Part model, mm, in its own coordinate system. A direction names the side the tool comes from. Coordinates: 2 decimals unless noted, no trailing zeros. Write each loop counter-clockwise with the first axis right and the second up, starting at its lowest first coordinate (ties: lowest second). Pieces come first, ordered by that corner, then holes. Notation, with made-up numbers: (33, 49) -> (63, 49) arc R29 cw to (63, 83) -> close; hole circle Ø7 at (10.25, 2). An arc over 180 degrees is marked (long way). Write item = value, one per line.
from build123d import *

# Parameters (mm, degrees)
SKETCH1_R           = 19.05
SKETCH1_R_2         = 9.525
BOSS_EXTRUDE1_DEPTH = 136.3472
SKETCH2_R           = 1.7526
CUT_EXTRUDE1_DEPTH  = 9.525
SKETCH3_R           = 1.7526
CUT_EXTRUDE2_DEPTH  = 9.525
SKETCH6_R           = 11.1125
CUT_EXTRUDE3_DEPTH  = 5.55625
SKETCH7_R           = 11.1125
CUT_EXTRUDE4_DEPTH  = 5.55625


with BuildPart() as part:
    # Sketch1 → Boss-Extrude1 (new body)
    with BuildSketch(Plane.XY):
        Circle(SKETCH1_R)
        Circle(SKETCH1_R_2, mode=Mode.SUBTRACT)
    extrude(amount=BOSS_EXTRUDE1_DEPTH)

    # Sketch2 → Cut-Extrude1 (cut)
    with BuildSketch(Plane(origin=(0, 0, 0), x_dir=(-1, 0, 0), z_dir=(0, 0, -1))):
        with Locations((0, 15.24)):
            Circle(SKETCH2_R)
        with Locations((15.24, 0)):
            Circle(SKETCH2_R)
        with Locations((0, -15.24)):
            Circle(SKETCH2_R)
        with Locations((-15.24, 0)):
            Circle(SKETCH2_R)
    extrude(amount=-CUT_EXTRUDE1_DEPTH, mode=Mode.SUBTRACT)

    # Sketch3 → Cut-Extrude2 (cut)
    with BuildSketch(Plane.XY.offset(136.3472)):
        with Locations((0, 15.24)):
            Circle(SKETCH3_R)
        with Locations((15.24, 0)):
            Circle(SKETCH3_R)
        with Locations((0, -15.24)):
            Circle(SKETCH3_R)
        with Locations((-15.24, 0)):
            Circle(SKETCH3_R)
    extrude(amount=-CUT_EXTRUDE2_DEPTH, mode=Mode.SUBTRACT)

    # Sketch6 → Cut-Extrude3 (cut)
    with BuildSketch(Plane.XY.offset(136.3472)):
        Circle(SKETCH6_R)
    extrude(amount=-CUT_EXTRUDE3_DEPTH, mode=Mode.SUBTRACT)

    # Sketch7 → Cut-Extrude4 (cut)
    with BuildSketch(Plane(origin=(0, 0, 0), x_dir=(-1, 0, 0), z_dir=(0, 0, -1))):
        Circle(SKETCH7_R)
    extrude(amount=-CUT_EXTRUDE4_DEPTH, mode=Mode.SUBTRACT)


solid = part.part
Q1. Saw through at C-C on y = 15.24. Give the cut face in (x, z) (3 decimals), and give its area (3 significant figures).
Model answer:
outline = (-11.43, 0) -> (-1.753, 0) -> (-1.753, 9.525) -> (1.753, 9.525) -> (1.753, 0) -> (11.43, 0) -> (11.43, 136.347) -> (1.753, 136.347) -> (1.753, 126.822) -> (-1.753, 126.822) -> (-1.753, 136.347) -> (-11.43, 136.347) -> close
area = 3,050 mm²
Q2. Pin check, flat tips, straight feed: pin 1 (3 mm diameter, centred on y = -2, z = 108.5, fed in from -X); pin 2 (2 mm diameter, centred on x = 0, y = -15.24, fed in from +Z); pin 3 (4 mm diameter, centred on y = -8.5, z = 46, fed in from -X). Stop position of each tip, or through.
Model answer:
pin_1 = -19.04
pin_2 = 126.82
pin_3 = -17.91
Q3. Mould opens along X. For faces 4 (the face through (16.99, 0.08, 4.7)), 5 (the face through (-15.12, -11.59, 67.22)), 6 (the face through (8, -8, 136.347)) say: released by +X, released by -X, zero draft, split by the parting line, or undercut.
Model answer:
face_4 = undercut
face_5 = split by the parting line
face_6 = zero draft
Q4. Probe line 1 (Y direction, x = 0, z = 135); line 2 (Y direction, x = 0.5, z = 87); line 3 (X direction, y = 3.5, z = 108.5). List the from-to ranges inside material, lowest first. Write a range as from..to.
Model answer:
line_1 = -19.05..-16.99, -13.49..-11.11, 11.11..13.49, 16.99..19.05
line_2 = -19.04..-9.51, 9.51..19.04
line_3 = -18.73..-8.86, 8.86..18.73
Q5. Which spindle directions (+Z, -Z, +X, -X, +Y, -Y) get a long thin tool onto all of the face, cutting with end or side? Do faces 1 (the face through (0, 15, 126.822)), 2 (the face through (8, -8, 0)), 3 (the face through (5, 8.3, 5.556)). Say none if no direction does.
Model answer:
face_1 = +Z
face_2 = -Z, +X, -X, +Y, -Y
face_3 = -Z
Q6. Saw through at A-A on y = 5. Give the cut face in (x, z).
Model answer:
outline = (-18.38, 0) -> (-9.92, 0) -> (-9.92, 5.56) -> (-8.11, 5.56) -> (-8.11, 130.79) -> (-9.92, 130.79) -> (-9.92, 136.35) -> (-18.38, 136.35) -> close; (8.11, 5.56) -> (9.92, 5.56) -> (9.92, 0) -> (18.38, 0) -> (18.38, 136.35) -> (9.92, 136.35) -> (9.92, 130.79) -> (8.11, 130.79) -> close
